```python
from build123d import *

# Parameters (mm, degrees)
F0_W     = 45.72
F0_H     = 6.35
F0_W_2   = 20.32
F0_H_2   = 34.987604
F1_DEPTH = 6.35
F3_DEPTH = 6.35
F5_DEPTH = 6.35


with BuildPart() as f1:
    # F0 (on Top) → F1 (new body)
    with BuildSketch(Plane.XY):
        Polygon((-22.86, 50.8), (-29.21, 50.8), (-29.21, 0), (-22.86, 0), (-22.86, 12.7), (-22.86, 19.05), align=None)
        Polygon((-22.86, 0), (-29.21, 0), (-16.51, -24.362533), (-16.51, -11.662533), align=None)
        with Locations((0, 15.875)):
            Rectangle(F0_W, F0_H)
        Polygon((-16.51, -11.662533), (-16.51, -24.362533), (-16.51, -59.350137), (16.51, -59.350137), (16.51, -24.362533), (16.51, -11.662533), align=None)
        with Locations((0, -35.506335)):
            Rectangle(F0_W_2, F0_H_2, mode=Mode.SUBTRACT)
        Polygon((22.86, 50.8), (22.86, 19.05), (22.86, 12.7), (22.86, 0), (29.21, 0), (29.21, 50.8), align=None)
        Polygon((22.86, 0), (16.51, -11.662533), (16.51, -24.362533), (29.21, 0), align=None)
    extrude(amount=F1_DEPTH)

    # F2 (on face) → F3 (join)
    with BuildSketch(Plane.YZ.offset(29.21)):
        with BuildLine():
            Line((50.8, 0), (38.1, 0))
            ThreePointArc((38.1, 0), (44.45, -6.35), (50.8, 0))
        make_face()
        with BuildLine():
            Line((12.7, 0), (0, 0))
            ThreePointArc((0, 0), (6.35, -6.35), (12.7, 0))
        make_face()
    extrude(amount=-F3_DEPTH)

    # F4 (on face) → F5 (join)
    with BuildSketch(Plane(origin=(-29.21, 0, 0), x_dir=(0, -1, 0), z_dir=(-1, 0, 0))):
        with BuildLine():
            Line((-38.1, 0), (-50.8, 0))
            ThreePointArc((-50.8, 0), (-44.45, -6.35), (-38.1, 0))
        make_face()
    extrude(amount=-F5_DEPTH)


solid = f1.part
```
Source: CAD feature listing. Evaluate the final solid. Frame: model axes, mm. A direction names the side the tool comes from. Round coordinates to 2 decimals unless told otherwise and drop trailing zeros. Write each loop counter-clockwise with the first axis right and the second up, starting at its lowest first coordinate (ties: lowest second). Pieces come first, ordered by that corner, then holes. Notation, with made-up numbers: M 71.25,49.5 L 89.25,49.5 A14 cw 89.25,58.5 Z; hole C 79,-3.75 d10. An arc over 180 degrees is marked long. Use CSV: the item, a comma, the result in double quotes. Start each with the question number.
Q1. Cut plane C-C on x = 3. Output: boundary loops of the cut face in (y, z), plus the area to 3 significant figures.
Q2. Access query for faces 5 (the face through (22.86, 38, 2)), 6 (the face through (0, -18.013, 3)), 7 (the face through (26.08, 6.21, -6.35)). Directions: +Z, -Z, +X, -X, +Y, -Y. A direction counts if a zero-diameter tool reaches every point of the face in a straight line with its end or side. Return the directions, or none.
Q3. First-contact query: P1, Ø3, axis at x = -3.5, z = 4, coming from the +Y side; P2, Ø10, axis at x = -19.5, y = -10, coming from the -Z side; P3, Ø5, axis at x = -18.5, z = 3.5, coming from the -Y side; P4, Ø5, axis at y = -40.5, z = 4.5, coming from the -X side. Flat tips, straight axial feed; report the tip coordinate or a pass-through.
Q4. Cut plane B-B on x = -15.5. Output: boundary loops of the cut face in (y, z).
Q5. Pull-direction query (Y, two-part tool) for faces 1 (the face through (26, 50.8, 3)), 2 (the face through (22.77, -12.35, 3.13)), 3 (the face through (29.21, 25, 2)), 4 (the face through (-10.16, -36, 3)); classes: +Y half, -Y half, draft (parallel to the pull), parting line (faces both ways), or undercut.
Q6. Line query: line 1 (Y direction, x = -4, z = 5); line 2 (X direction, y = 0.5, z = 4); line 3 (Y direction, x = -16, z = 4.5). Output: solid intervals per line, ascending. Write a range as from..to.
Q7. Cut plane D-D on z = 4. Output: boundary loops of the cut face in (x, y), plus the area to 3 significant figures.
Q8. Cut plane A-A on y = -30. Output: boundary loops of the cut face in (x, z).
Results found:
1,outline,"M -59.35,0 L -53,0 L -53,6.35 L -59.35,6.35 Z; M -18.01,0 L -11.66,0 L -11.66,6.35 L -18.01,6.35 Z; M 12.7,0 L 19.05,0 L 19.05,6.35 L 12.7,6.35 Z"
1,area,"121 mm^2"
2,face 5,"+Z, -Z, +Y"
2,face 6,"+Z, -Z"
2,face 7,"-Z, +X, -X"
3,P1,"y = 19.05"
3,P2,"z = 0"
3,P3,"y = -59.35"
3,P4,"x = -16.51"
4,outline,"M -59.35,0 L -11.66,0 L -11.66,6.35 L -59.35,6.35 Z; M 12.7,0 L 19.05,0 L 19.05,6.35 L 12.7,6.35 Z"
5,face 1,"+Y half"
5,face 2,"-Y half"
5,face 3,"draft"
5,face 4,"undercut"
6,line 1,"-59.35..-53, -18.01..-11.66, 12.7..19.05"
6,line 2,"-29.21..-22.86, 22.86..29.21"
6,line 3,"-59.35..-11.66, 12.7..19.05"
7,outline,"M -29.21,0 L -16.51,-24.36 L -16.51,-59.35 L 16.51,-59.35 L 16.51,-24.36 L 29.21,0 L 29.21,50.8 L 22.86,50.8 L 22.86,19.05 L -22.86,19.05 L -22.86,50.8 L -29.21,50.8 Z; hole M -22.86,0 L -16.51,-11.66 L 16.51,-11.66 L 22.86,0 L 22.86,12.7 L -22.86,12.7 Z; hole M -10.16,-53 L 10.16,-53 L 10.16,-18.01 L -10.16,-18.01 Z"
7,area,"2,030 mm^2"
8,outline,"M -16.51,0 L -10.16,0 L -10.16,6.35 L -16.51,6.35 Z; M 10.16,0 L 16.51,0 L 16.51,6.35 L 10.16,6.35 Z"
